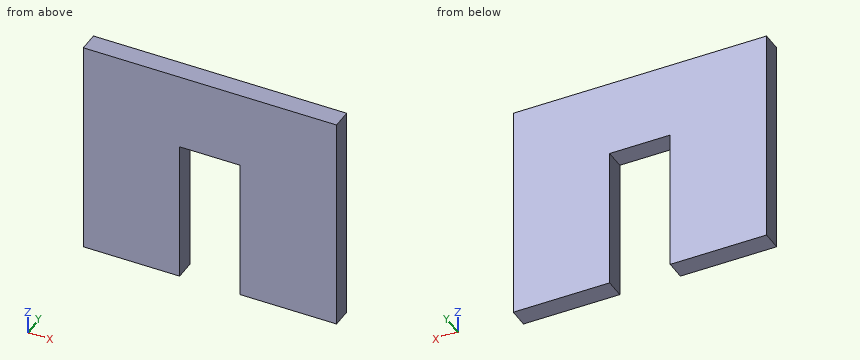
Autodesk Inventor part; units mm, degrees
ref_plane "YZ Plane" through (0, 0, 0) normal (1, 0, 0) x (0, 1, 0)
ref_plane "XZ Plane" through (0, 0, 0) normal (0, 1, 0) x (-1, 0, 0)
ref_plane "XY Plane" through (0, 0, 0) normal (0, 0, 1) x (1, 0, 0)
sketch "Sketch1" plane through (0, 0, 0) normal (0, 1, 0) x (-1, 0, 0)
  line L0 (0.2295, -3) -> (23.2295, -3)
  line L1 (23.2295, -3) -> (23.2295, -23)
  line L2 (0.2295, -23) -> (0.2295, -3)
  line L3 (8.9795, -23) -> (8.9795, -10)
  line L4 (8.9795, -10) -> (14.4795, -10)
  line L5 (14.4795, -10) -> (14.4795, -23)
  line L6 (11.7295, -5) -> (11.7295, -18.3097) construction
  line L7 (23.2295, -23) -> (14.4795, -23)
  line L8 (8.9795, -23) -> (0.2295, -23)
  dimension "d4" = 23
  dimension "d5" = 20
  dimension "d8" = 5.5
  dimension "d9" = 13
extrude "Extrusion1" add sketch "Sketch1" along normal blind 1.8
properties part number "Distance_test_rig_insert"
Geometry check sheet. Reference: the model listing, model coordinates, mm. Give positions to 0.01 mm unless a question says otherwise; leave off trailing zeros. Order: outer loops, then holes, each group sorted by start corner. A loop starts at its lowest first (then second) coordinate and runs counter-clockwise, first axis right, second up.
1. Sectioned sample at A-A (z = -18.75). Record the boundary of the cut face in (x, y).
Completed:
outline: (-23.23, 0) - (-14.48, 0) - (-14.48, 1.8) - (-23.23, 1.8) - close; (-8.98, 0) - (-0.23, 0) - (-0.23, 1.8) - (-8.98, 1.8) - close
2. Scan lines: line 1 (X direction, y = 1.15, z = -20.25); line 2 (Z direction, x = -12.75, y = 0.6). Record each from-to range of solid material in increasing order.
Completed:
line 1: x = -23.23 to -14.48, -8.98 to -0.23
line 2: z = -10 to -3
3. Depth check by flat-ended pin: pin 1 (1 mm diameter, centred on x = -12, z = -15, fed in from +Y). Enter the tip coordinate at first touch or a pass-through.
Completed:
pin 1: passes through
4. Sectioned sample at B-B (y = 1.35). Record the boundary of the cut face in (x, z).
Completed:
outline: (-23.23, -23) - (-14.48, -23) - (-14.48, -10) - (-8.98, -10) - (-8.98, -23) - (-0.23, -23) - (-0.23, -3) - (-23.23, -3) - close
